CAD build for the part. Positions are in the model's coordinates, mm. Face numbers are marked on the shaded views. A direction names the side the tool comes from. Coordinates: 2 decimals unless noted, no trailing zeros. Write each loop counter-clockwise with the first axis right and the second up, starting at its lowest first coordinate (ties: lowest second). Pieces come first, ordered by that corner, then holes.
```python
from build123d import *

# Parameters (mm, degrees)
ESQUISSE1_W                                    = 49.2
ESQUISSE1_H                                    = 52
BOSS_EXTRU_1_DEPTH                             = 40
COQUE1_T                                       = 4
CONG_1_R                                       = 2
CONG_2_R                                       = 2
CONG_3_R                                       = 2
CONG_4_R                                       = 2
ESQUISSE5_R                                    = 1.8
BOSS_EXTRU_2_DEPTH                             = 9
ESQUISSE9_W                                    = 4
ESQUISSE9_H                                    = 15.843796137
ENL_V_MAT_EXTRU_3_DEPTH                        = 36
ESQUISSE11_W                                   = 8.5
ESQUISSE11_H                                   = 8.5
BOSS_EXTRU_4_DEPTH                             = 7
CONG_5_R                                       = 4
CONG_6_R                                       = 4
CONG_7_R                                       = 1
CONG_8_R                                       = 1
FRAISAGE_POUR_VIS_T_TE_FRAIS_E_M31_D           = 3.4
FRAISAGE_POUR_VIS_T_TE_FRAIS_E_M31_CSINK_D     = 6.3
FRAISAGE_POUR_VIS_T_TE_FRAIS_E_M31_CSINK_ANGLE = 90


with BuildPart() as part:
    # Esquisse1 → Boss.-Extru.1 (new body)
    with BuildSketch(Plane(origin=(0, 0, 0), x_dir=(1, 0, 0), z_dir=(0, 1, 0))):
        Rectangle(ESQUISSE1_W, ESQUISSE1_H)
    extrude(amount=BOSS_EXTRU_1_DEPTH)

    # Coque1
    coque1_openings = [part.faces().sort_by_distance(p)[0] for p in [
        (0, 40, 0),
    ]]
    offset(amount=COQUE1_T, openings=coque1_openings, kind=Kind.INTERSECTION)

    # Congé1
    # the kernel refuses this fillet: 2 mm, written as the material it takes off along each edge
    with BuildSketch(Plane(origin=(28.6, -9, 30), x_dir=(-1, 0, 0), z_dir=(0, 1, 0))) as cong_1_piece_1:
        with BuildLine():
            CenterArc((CONG_1_R, -CONG_1_R), CONG_1_R, 90, 90)
            Line((0, -CONG_1_R), (0, 0))
            Line((0, 0), (CONG_1_R, 0))
        make_face()
    extrude(amount=54, mode=Mode.SUBTRACT)

    # Congé2
    cong_2_edges = [part.edges().sort_by_distance(p)[0] for p in [
        (28.6, 18, -30),
    ]]
    fillet(cong_2_edges, radius=CONG_2_R)

    # Congé3
    cong_3_edges = [part.edges().sort_by_distance(p)[0] for p in [
        (-28.6, 18, -30),
    ]]
    fillet(cong_3_edges, radius=CONG_3_R)

    # Congé4
    cong_4_edges = [part.edges().sort_by_distance(p)[0] for p in [
        (-28.6, 18, 30),
    ]]
    fillet(cong_4_edges, radius=CONG_4_R)

    # Esquisse5 → Boss.-Extru.2 (add)
    with BuildSketch(Plane(origin=(0, 0, 0), x_dir=(1, 0, 0), z_dir=(0, 1, 0))):
        with Locations(Location((-22.6, -2.6, 0), (0, 0, 90))):
            Circle(ESQUISSE5_R)
        with Locations(Location((22.6, -2.6, 0), (0, 0, 90))):
            Circle(ESQUISSE5_R)
        with Locations(Location((-22.6, -24, 0), (0, 0, 90))):
            Circle(ESQUISSE5_R)
        with Locations(Location((22.6, -24, 0), (0, 0, 90))):
            Circle(ESQUISSE5_R)
    extrude(amount=BOSS_EXTRU_2_DEPTH)

    # Esquisse9 → Enlèv. mat.-Extru.3 (cut)
    with BuildSketch(Plane(origin=(0, 40, 0), x_dir=(1, 0, 0), z_dir=(0, 1, 0))):
        with Locations((26.6, -12.636910853)):
            Rectangle(ESQUISSE9_W, ESQUISSE9_H)
    extrude(amount=-ENL_V_MAT_EXTRU_3_DEPTH, mode=Mode.SUBTRACT)

    # Esquisse11 → Boss.-Extru.4 (add)
    with BuildSketch(Plane(origin=(0, -4, 0), x_dir=(-1, 0, 0), z_dir=(0, -1, 0))):
        with Locations((32.85, 19.732237021)):
            Rectangle(ESQUISSE11_W, ESQUISSE11_H)
        with Locations((-32.85, 19.732237021)):
            Rectangle(ESQUISSE11_W, ESQUISSE11_H)
    extrude(amount=-BOSS_EXTRU_4_DEPTH)

    # Congé5
    cong_5_edges = [part.edges().sort_by_distance(p)[0] for p in [
        (37.1, -0.5, -15.482237021),
        (37.1, -0.5, -23.982237021),
    ]]
    fillet(cong_5_edges, radius=CONG_5_R)

    # Congé6
    cong_6_edges = [part.edges().sort_by_distance(p)[0] for p in [
        (-37.1, -0.5, -23.982237021),
        (-37.1, -0.5, -15.482237021),
    ]]
    fillet(cong_6_edges, radius=CONG_6_R)

    # Congé7
    cong_7_edges = [part.edges().sort_by_distance(p)[0] for p in [
        (-37.1, 3, -19.732237021),
        (-30.85, 3, -23.982237021),
        (-35.928427125, 3, -16.653809897),
        (-35.928427125, 3, -22.810664146),
        (-30.85, 3, -15.482237021),
    ]]
    fillet(cong_7_edges, radius=CONG_7_R)

    # Congé8
    cong_8_edges = [part.edges().sort_by_distance(p)[0] for p in [
        (37.1, 3, -19.732237021),
        (30.85, 3, -15.482237021),
        (35.928427125, 3, -22.810664146),
        (35.928427125, 3, -16.653809897),
        (30.85, 3, -23.982237021),
    ]]
    fillet(cong_8_edges, radius=CONG_8_R)

    # Fraisage pour vis à tête fraisée M31 (through all)
    with Locations(Plane(origin=(0, 3, 0), x_dir=(1, 0, 0), z_dir=(0, 1, 0))):
        with Locations((-32.904561285, 19.825700849), (32.940796686, 19.825700849)):
            CounterSinkHole(FRAISAGE_POUR_VIS_T_TE_FRAIS_E_M31_D / 2, FRAISAGE_POUR_VIS_T_TE_FRAIS_E_M31_CSINK_D / 2, counter_sink_angle=FRAISAGE_POUR_VIS_T_TE_FRAIS_E_M31_CSINK_ANGLE)


solid = part.part
```
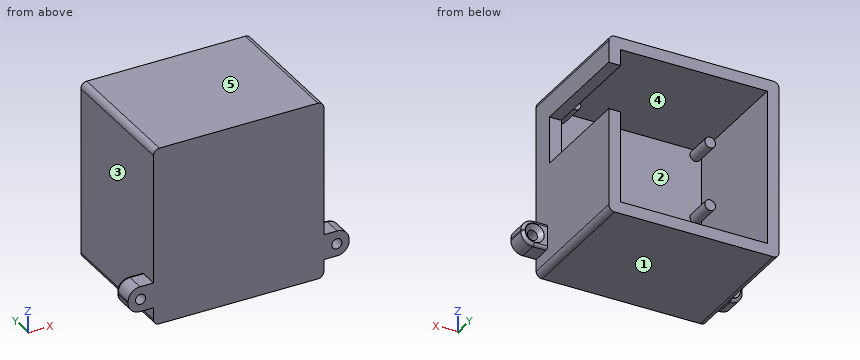
Item 1: Flat gauge pins, fed straight in: pin 1 Ø12 at (y, z) = (26.5, -3) entering from +X; pin 2 Ø2 at (x, y) = (-31.5, 0) entering from -Z; pin 3 Ø15 at (x, z) = (8, -12) entering from +Y. Where does each tip first touch, or does it go through?
Item 2: Two-plate mould, pull along X, no slides. Class the marked faces 1, 2 and 3: +X half, -X half, draft (parallel to the pull), parting line (faces both ways), or undercut.
Item 3: Saw through at B-B, the plane x = -22.6. Write the cut outline in (y, z).
Item 4: Which spindle directions (+Z, -Z, +X, -X, +Y, -Y) get a long thin tool onto all of the face, cutting with end or side? Do the marked faces 4 and 5. Say none if no direction does.
Item 5: Wall check: line 1 along Z through (x, y) = (6, 21.5); line 2 along X through (y, z) = (2, 6); line 3 along X through (y, z) = (10, 10.5). Give the ranges that are in metal, low to high.
Item 6: Saw through at A-A, the plane z = 2.6. Write the cut outline in (x, y).
Item 7: Saw through at D-D, the plane x = -9.5. Write the cut outline in (y, z), and give its area (3 significant figures).
Item 8: Saw through at C-C, the plane z = 15.5. Write the cut outline in (x, y).
Working result:
1. pin 1: stops at x = 28.6
1. pin 2: stops at z = -23.98
1. pin 3: stops at y = 0
2. face 1: draft
2. face 2: undercut
2. face 3: -X half
3. outline: (-4, -30) - (40, -30) - (40, -26) - (0, -26) - (0, 0.8) - (9, 0.8) - (9, 4.4) - (0, 4.4) - (0, 22.2) - (9, 22.2) - (9, 25.8) - (0, 25.8) - (0, 26) - (40, 26) - (40, 30) - (-4, 30) - close
4. face 4: +Y
4. face 5: +Z, +X, -X, +Y, -Y
5. line 1: z = -30 to -26, 26 to 30
5. line 2: x = -28.6 to -24.6, 24.6 to 28.6
5. line 3: x = -28.6 to -24.6
6. outline: (-28.6, -4) - (28.6, -4) - (28.6, 40) - (24.6, 40) - (24.6, 0) - (24.4, 0) - (24.4, 9) - (20.8, 9) - (20.8, 0) - (-20.8, 0) - (-20.8, 9) - (-24.4, 9) - (-24.4, 0) - (-24.6, 0) - (-24.6, 40) - (-28.6, 40) - close
7. outline: (-4, -30) - (40, -30) - (40, -26) - (0, -26) - (0, 26) - (40, 26) - (40, 30) - (-4, 30) - close
7. area: 560 mm2
8. outline: (-28.6, -4) - (28.6, -4) - (28.6, 4) - (24.6, 4) - (24.6, 0) - (-24.6, 0) - (-24.6, 40) - (-28.6, 40) - close
